Study the drawing (mm; zero at the part's minimum x, y, z) and answer. A direction names the side the tool comes from. Give positions to 0.01 mm unless a question says otherwise; leave off trailing zeros. Write each loop counter-clockwise with the first axis right and the second up, starting at its lowest first coordinate (ties: lowest second). Pieces come first, ordered by that corner, then holes.
1) Find section D-D (y = 3). Determine the outline of the cut face in (x, z).
2) Given pin 1 Ø1 at (y, z) = (5.5, 25.5) entering from -X; pin 2 Ø6 at (x, y) = (51.5, 16) entering from +Z; pin 3 Ø10 at (x, z) = (25.5, 14.5) entering from +Y, each flat-ended and moving along its own axis, determine where each tip first touches the part or whether it passes through.
3) Straight lines are drawn through the part: probe 1 along Y at (x, z) = (35, 2.75); probe 2 along X at (y, z) = (10, 27.75); probe 3 along X at (y, z) = (2.75, 27.5). For each, find the intervals that lie inside material, in ascending order.
4) Find section B-B (x = 35). Determine the outline of the cut face in (y, z), plus the area to 3 significant figures.
5) Find section A-A (z = 8.5). Determine the outline of the cut face in (x, y).
6) Determine the mould class of the marked faces 1, 2 and 3 for opening direction X: pulls with the +X half, pulls with the -X half, needs draft (parallel to the pull), parting line crosses it, or undercut.
7) A tool of negligible diameter and unlimited length cuts with its end or side. For the marked faces 4, 5 and 6, from which of +Z, -Z, +X, -X, +Y, -Y can it reach the whole face along a straight path? Write none if from no direction.
8) Find section C-C (x = 64). Determine the outline of the cut face in (y, z).
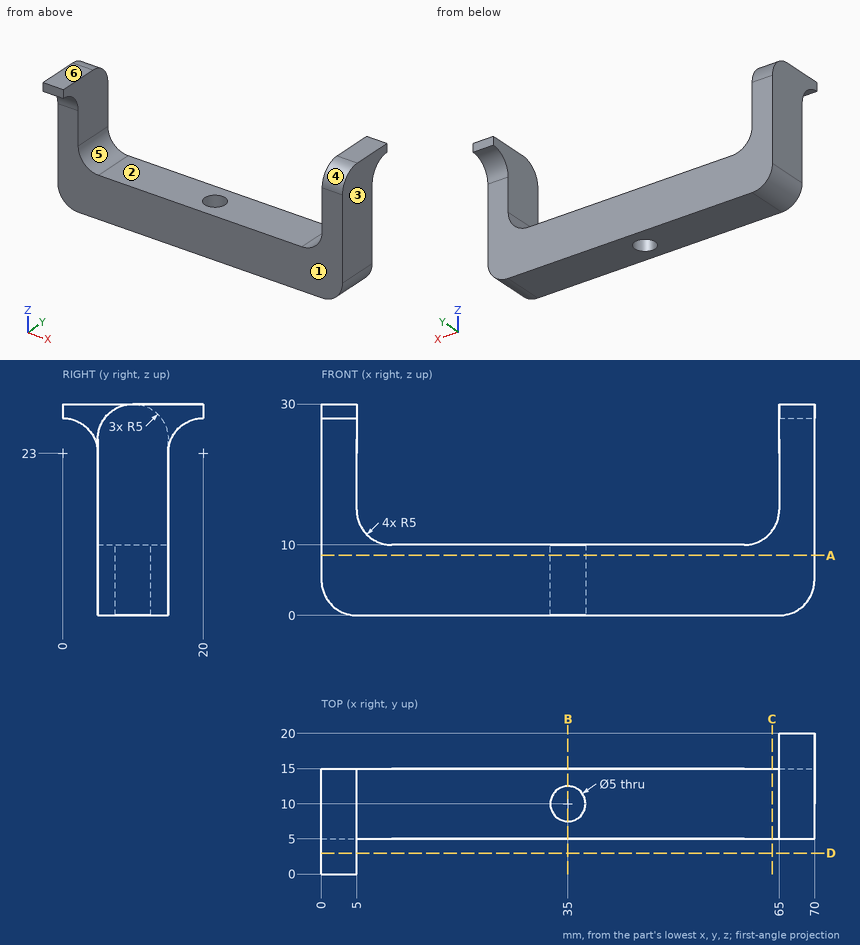
Results:
1. outline: (0, 27) - (5, 27) - (5, 30) - (0, 30) - close
2. pin 1: stops at x = 0
2. pin 2: stops at z = 10
2. pin 3: stops at y = 15
3. probe 1: y = 5 to 7.5, 12.5 to 15
3. probe 2: x = 0 to 5, 65 to 70
3. probe 3: x = 0 to 5
4. outline: (5, 0) - (7.5, 0) - (7.5, 10) - (5, 10) - close; (12.5, 0) - (15, 0) - (15, 10) - (12.5, 10) - close
4. area: 50.0 mm2
5. outline: (0, 5) - (70, 5) - (70, 15) - (0, 15) - close; hole circle Ø5 at (35, 10)
6. face 1: needs draft
6. face 2: undercut
6. face 3: pulls with the +X half
7. face 4: +Z, +X, -Y
7. face 5: +Z, +Y, -Y
7. face 6: +Z, +X, -X, +Y, -Y
8. outline: (5, 0) - (15, 0) - (15, 12) - (5, 12) - close
